Source: CAD feature listing. Evaluate the final solid. Frame: model axes, mm. Give positions to 0.01 mm unless a question says otherwise; leave off trailing zeros. Order: outer loops, then holes, each group sorted by start corner. A loop starts at its lowest first (then second) coordinate and runs counter-clockwise, first axis right, second up. Notation, with made-up numbers: M 73,-29 L 124,-29 A32 cw 124,0 Z; hole C 52.5,32 d5. An arc over 180 degrees is marked long. Answer in a Markdown table with one row per item. Add a question column.
(1) Section query A-A, the plane y = -66. Return loops of the section in (x, z).
(2) Pin query (flat end, axial travel): P1, Ø1, axis at x = 23, z = 2.5, coming from the +Y side; P2, Ø1, axis at y = 8.5, z = 0.5, coming from the +X side. Return the tip coordinate at first contact, or that it passes through.
(3) Material intervals for line 1 along X through (y, z) = (8, 0.45); line 2 along Y through (x, z) = (30, 2.4); line 3 along X through (y, z) = (-66, 0.9), sorted ascending.
(4) Mould query, pull axis X, two halves, no side actions, for faces 1 (the face through (1, -31, 3)), 2 (the face through (-70, -29, 1)), 3 (the face through (54.964, -82.242, 1.479)). Classes: pulls with the +X half, pulls with the -X half, needs draft (parallel to the pull), parting line crosses it, or undercut.
from build123d import *

# Parameters (mm, degrees)
BOSS_EXTRUDE1_DEPTH = 3


with BuildPart() as part:
    # Sketch1 → Boss-Extrude1 (new body)
    with BuildSketch(Plane.XY):
        with BuildLine():
            add(Edge.make_bspline(
                [(-70, -11.5), (-70, 26.5), (-18, 33.5), (-10, 33.5)],
                knots=[0, 0, 0, 0, 1, 1, 1, 1], degree=3))
            Line((-70, -11.5), (-70, -46.5))
            ThreePointArc((-70, -46.5), (-55.355339059, -81.855339059), (-20, -96.5))
            Line((-20, -96.5), (20, -96.5))
            ThreePointArc((20, -96.5), (55.355339059, -81.855339059), (70, -46.5))
            Line((70, -46.5), (70, -11.5))
            add(Edge.make_bspline(
                [(10, 33.5), (18, 33.5), (70, 26.5), (70, -11.5)],
                knots=[0, 0, 0, 0, 1, 1, 1, 1], degree=3))
            Line((10, 33.5), (-10, 33.5))
        make_face()
    extrude(amount=BOSS_EXTRUDE1_DEPTH)


solid = part.part
Values follow:
| question | item | result |
|---|---|---|
| 1 | outline | M -66.04,0 L 66.04,0 L 66.04,3 L -66.04,3 Z |
| 2 | P1 | stops at y = 31.86 |
| 2 | P2 | stops at x = 64.38 |
| 3 | line 1 | x = -64.38 to 64.38 |
| 3 | line 2 | y = -95.49 to 30.03 |
| 3 | line 3 | x = -66.04 to 66.04 |
| 4 | face 1 | needs draft |
| 4 | face 2 | pulls with the -X half |
| 4 | face 3 | pulls with the +X half |
